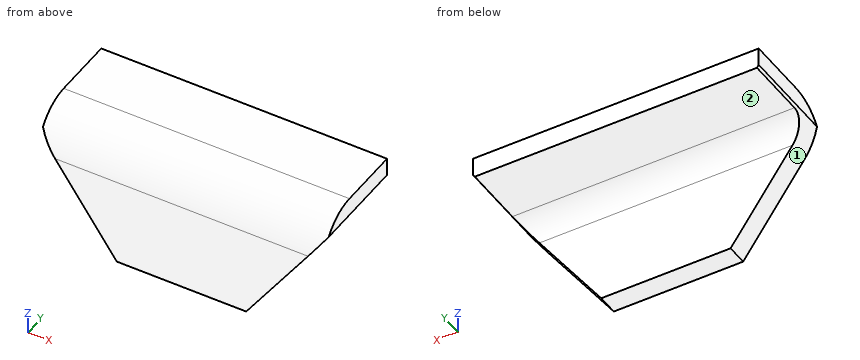
from build123d import *

# Parameters (mm, degrees)
SKETCH1_W                    = 110
SKETCH1_H                    = 50
BASE_FLANGE1_DEPTH           = 8
EDGE_FLANGE1_STRIP_W         = 48
EDGE_FLANGE1_STRIP_H         = 8
EDGE_FLANGE1_STRIP_CUT_DEPTH = 110
EDGE_FLANGE1_DEPTH           = 110
CHAMFER1_SIZE                = 43
CHAMFER1_SIZE2               = 30.108924143
MIRROR2_START                = 34.728986582
MIRROR2_OUTLINE_W            = 56
MIRROR2_OUTLINE_H            = 41
MIRROR2_DEPTH                = 24.663786763


# Read off the part's stored shape, not the designer's step: Mirror2
# Sheet-metal steps are written as plain solids
with BuildPart() as part:
    # Sketch1 → Base-Flange1 (new body)
    with BuildSketch(Plane(origin=(0, 0, 0), x_dir=(1, 0, 0), z_dir=(0, 1, 0))):
        Rectangle(SKETCH1_W, SKETCH1_H)
    extrude(amount=-BASE_FLANGE1_DEPTH)

    # Edge-Flange1 strip (across the edge) → Edge-Flange1 strip cut (cut)
    with BuildSketch(Plane(origin=(-55, 0, 25), x_dir=(0, 0, -1), z_dir=(1, 0, 0))):
        with Locations((-8, -4)):
            Rectangle(EDGE_FLANGE1_STRIP_W, EDGE_FLANGE1_STRIP_H)
    extrude(amount=EDGE_FLANGE1_STRIP_CUT_DEPTH, mode=Mode.SUBTRACT)

    # Edge-Flange1 section (across the edge) → Edge-Flange1 (add)
    with BuildSketch(Plane(origin=(-55, 0, 25), x_dir=(0, 0, -1), z_dir=(1, 0, 0))):
        with BuildLine():
            Line((0, 8), (0, 32))
            Line((0, 32), (8, 32))
            Line((8, 32), (8, 8))
            ThreePointArc((8, 8), (10.343145751, 2.343145751), (16, 0))
            Line((16, 0), (16, -8))
            ThreePointArc((16, -8), (4.686291501, -3.313708499), (0, 8))
        make_face()
    extrude(amount=EDGE_FLANGE1_DEPTH)

    # Chamfer1
    chamfer1_edges = [part.edges().sort_by_distance(p)[0] for p in [
        (-55, -4, -25),
    ]]
    chamfer1_side = [part.faces().sort_by_distance(p)[0] for p in [
        (-55, -0.640312424, -8),
    ]]
    chamfer(chamfer1_edges, length=CHAMFER1_SIZE, length2=CHAMFER1_SIZE2, reference=chamfer1_side[0])

    # Mirror2 outline → Mirror2 (cut)
    with BuildSketch(Plane(origin=(0, 0, 0), x_dir=(0.5735764363510512, 0, 0.8191520442889882), z_dir=(0.8191520442889882, 0, -0.5735764363510512)).offset(MIRROR2_START)):
        with Locations((20, -12.5)):
            Rectangle(MIRROR2_OUTLINE_W, MIRROR2_OUTLINE_H)
    extrude(amount=MIRROR2_DEPTH, mode=Mode.SUBTRACT)


solid = part.part
The listing builds one solid part. Answer for the finished solid, in the listing's coordinates (mm). Face numbers are marked on the shaded views. A direction names the side the tool comes from. Coordinates: 2 decimals unless noted, no trailing zeros. Write each loop counter-clockwise with the first axis right and the second up, starting at its lowest first coordinate (ties: lowest second). Pieces come first, ordered by that corner, then holes. Notation, with made-up numbers: (-11.5, 1) - (-0.5, 1) arc R25 cw to (-0.5, 32) - close; hole circle Ø5 at (71.25, 40). An arc over 180 degrees is marked (long way). Answer as CSV lines item,"result".
1. Find section C-C (z = -16.5). Give the vertices of the cut face in (x, y), plus the area to 3 significant figures.
Computed values:
outline,"(-30.84, -8) - (30.84, -8) - (30.84, 0) - (-30.84, 0) - close"
area,"493 mm²"
2. A tool of negligible diameter and unlimited length cuts with its end or side. For the marked faces 1 and 2, from which of +Z, -Z, +X, -X, +Y, -Y can it reach the whole face along a straight path? Write none if from no direction.
Computed values:
face 1,"-Z, -X, +Y, -Y"
face 2,"-Z, +X, -X, +Y"
3. Given P1, Ø1, axis at x = 20, y = 26, coming from the -Z side; P2, Ø10, axis at x = -13, z = 8, coming from the +Y side; P3, Ø3, axis at x = 10.5, z = -2, coming from the +Y side, each flat-ended and moving along its own axis, determine where each tip first touches the part or whether it passes through.
Computed values:
P1,"stops at z = 17"
P2,"stops at y = 1.07"
P3,"stops at y = 0"
4. Find section D-D (x = -31.5). Give the vertices of the cut face in (y, z).
Computed values:
outline,"(-8, -15.56) - (0, -15.56) - (0, 9) arc R8 cw to (8, 17) - (32, 17) - (32, 25) - (8, 25) arc R16 ccw to (-8, 9) - close"
5. Straight lines are drawn through the part: line 1 (Z direction, x = 50, y = 23); line 2 (Y direction, x = 30, z = 9); line 3 (Y direction, x = -18, z = 14.5). For each, find the intervals that lie inside material, in ascending order. Write a range as [from, to].
Computed values:
line 1,"z = [17, 25]"
line 2,"y = [-8, 0]"
line 3,"y = [-7.02, 2.19]"
6. Find section B-B (y = 18.5). Give the vertices of the cut face in (x, z), plus the area to 3 significant figures.
Computed values:
outline,"(-55, 18) - (-54.3, 17) - (54.3, 17) - (55, 18) - (55, 25) - (-55, 25) - close"
area,"879 mm²"
7. Find section A-A (x = -12.5). Give the vertices of the cut face in (y, z), plus the area to 3 significant figures.
Computed values:
outline,"(-8, -25) - (0, -25) - (0, 9) arc R8 cw to (8, 17) - (32, 17) - (32, 25) - (8, 25) arc R16 ccw to (-8, 9) - close"
area,"615 mm²"
